Read the model definition and answer for the solid it produces. Units are mm, in the model's axes. Face numbers are marked on the shaded views. Coordinates: 2 decimals unless noted, no trailing zeros. Loops run counter-clockwise (first coordinate to the right, second up) from the corner with the lowest first, then second, coordinate; pieces in that order, holes last.
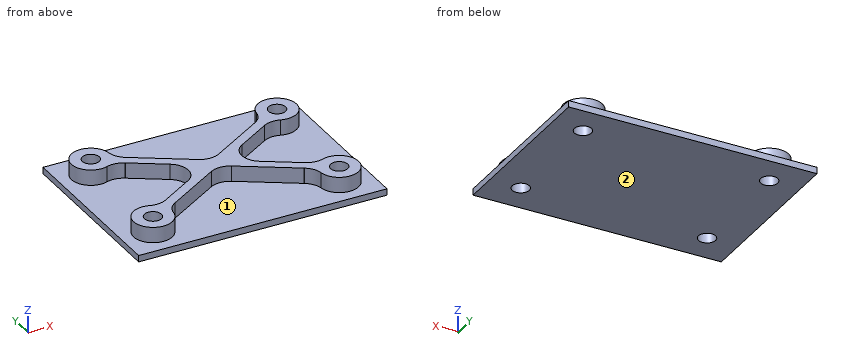
from build123d import *

# Parameters (mm, degrees)
F1_DEPTH = 3.175
F3_DEPTH = 7.62
F4_R     = 9.525
F5_R     = 4.2037
F6_DEPTH = 10.796


with BuildPart() as f1:
    # F0 (on Top) → F1 (new body)
    with BuildSketch(Plane.XY):
        with BuildLine():
            Line((15.24, -56.515), (15.24, 0))
            ThreePointArc((15.24, 0), (-10.7763073453, -10.7763073453), (0, 15.24))
            Line((0, 15.24), (-91.44, 15.24))
            ThreePointArc((-91.44, 15.24), (-80.6636926547, 10.7763073453), (-76.2, 0))
            ThreePointArc((-76.2, 0), (-91.44, -15.24), (-106.68, 0))
            Line((-106.68, 0), (-106.68, -56.515))
            ThreePointArc((-106.68, -56.515), (-91.44, -41.275), (-76.2, -56.515))
            ThreePointArc((-76.2, -56.515), (-80.6636926547, -67.2913073453), (-91.44, -71.755))
            Line((-91.44, -71.755), (0, -71.755))
            ThreePointArc((0, -71.755), (-10.7763073453, -45.7386926547), (15.24, -56.515))
        make_face()
        with BuildLine():
            ThreePointArc((-106.68, -56.515), (-102.2163073453, -67.2913073453), (-91.44, -71.755))
            ThreePointArc((-91.44, -71.755), (-80.6636926547, -67.2913073453), (-76.2, -56.515))
            ThreePointArc((-76.2, -56.515), (-91.44, -41.275), (-106.68, -56.515))
        make_face()
        with BuildLine():
            ThreePointArc((-76.2, 0), (-80.6636926547, 10.7763073453), (-91.44, 15.24))
            ThreePointArc((-91.44, 15.24), (-102.2163073453, 10.7763073453), (-106.68, 0))
            ThreePointArc((-106.68, 0), (-91.44, -15.24), (-76.2, 0))
        make_face()
        with BuildLine():
            ThreePointArc((0, 15.24), (-10.7763073453, -10.7763073453), (15.24, 0))
            ThreePointArc((15.24, 0), (10.7763073453, 10.7763073453), (0, 15.24))
        make_face()
        with BuildLine():
            ThreePointArc((0, -71.755), (10.7763073453, -67.2913073453), (15.24, -56.515))
            ThreePointArc((15.24, -56.515), (-10.7763073453, -45.7386926547), (0, -71.755))
        make_face()
        with BuildLine():
            Line((15.24, -71.755), (15.24, -56.515))
            ThreePointArc((15.24, -56.515), (10.7763073453, -67.2913073453), (0, -71.755))
            Line((0, -71.755), (15.24, -71.755))
        make_face()
        with BuildLine():
            Line((-106.68, -71.755), (-91.44, -71.755))
            ThreePointArc((-91.44, -71.755), (-102.2163073453, -67.2913073453), (-106.68, -56.515))
            Line((-106.68, -56.515), (-106.68, -71.755))
        make_face()
        with BuildLine():
            ThreePointArc((-106.68, 0), (-102.2163073453, 10.7763073453), (-91.44, 15.24))
            Line((-91.44, 15.24), (-106.68, 15.24))
            Line((-106.68, 15.24), (-106.68, 0))
        make_face()
        with BuildLine():
            ThreePointArc((0, 15.24), (10.7763073453, 10.7763073453), (15.24, 0))
            Line((15.24, 0), (15.24, 15.24))
            Line((15.24, 15.24), (0, 15.24))
        make_face()
    extrude(amount=-F1_DEPTH)

    # F2 (on face) → F3 (join)
    with BuildSketch(Plane.XY):
        with BuildLine():
            Line((-9.0970156165, -2.8231067769), (-14.056494823, -5.8883404532))
            ThreePointArc((-14.056494823, -5.8883404532), (-12.9637932823, -8.0123444592), (-11.5526371794, -9.9395258539))
            Line((-11.5526371794, -9.9395258539), (-6.593157973, -6.8742921776))
            ThreePointArc((-6.593157973, -6.8742921776), (8.1023708015, 5.007715287), (-9.0970156165, -2.8231067769))
        make_face()
        with BuildLine():
            ThreePointArc((-11.5526371794, -46.5754741461), (-12.9637932823, -48.5026555408), (-14.056494823, -50.6266595468))
            Line((-14.056494823, -50.6266595468), (-9.0970156165, -53.6918932231))
            ThreePointArc((-9.0970156165, -53.6918932231), (8.1023708015, -61.522715287), (-6.593157973, -49.6407078224))
            Line((-6.593157973, -49.6407078224), (-11.5526371794, -46.5754741461))
        make_face()
        with BuildLine():
            ThreePointArc((-77.383505177, -50.6266595468), (-78.4762067177, -48.5026555408), (-79.8873628206, -46.5754741461))
            Line((-79.8873628206, -46.5754741461), (-84.846842027, -49.6407078224))
            ThreePointArc((-84.846842027, -49.6407078224), (-99.5423708015, -61.522715287), (-82.3429843835, -53.6918932231))
            Line((-82.3429843835, -53.6918932231), (-77.383505177, -50.6266595468))
        make_face()
        with BuildLine():
            ThreePointArc((-82.3429843835, -2.8231067769), (-99.5423708015, 5.007715287), (-84.846842027, -6.8742921776))
            Line((-84.846842027, -6.8742921776), (-79.8873628206, -9.9395258539))
            ThreePointArc((-79.8873628206, -9.9395258539), (-78.4762067177, -8.0123444592), (-77.383505177, -5.8883404532))
            Line((-77.383505177, -5.8883404532), (-82.3429843835, -2.8231067769))
        make_face()
        with BuildLine():
            ThreePointArc((-77.383505177, -5.8883404532), (-78.4762067177, -8.0123444592), (-79.8873628206, -9.9395258539))
            Line((-79.8873628206, -9.9395258539), (-50.249292292, -28.2575))
            Line((-50.249292292, -28.2575), (-79.8873628206, -46.5754741461))
            ThreePointArc((-79.8873628206, -46.5754741461), (-78.4762067177, -48.5026555408), (-77.383505177, -50.6266595468))
            Line((-77.383505177, -50.6266595468), (-45.72, -31.0568542638))
            Line((-45.72, -31.0568542638), (-14.056494823, -50.6266595468))
            ThreePointArc((-14.056494823, -50.6266595468), (-12.9637932823, -48.5026555408), (-11.5526371794, -46.5754741461))
            Line((-11.5526371794, -46.5754741461), (-41.190707708, -28.2575))
            Line((-41.190707708, -28.2575), (-11.5526371794, -9.9395258539))
            ThreePointArc((-11.5526371794, -9.9395258539), (-12.9637932823, -8.0123444592), (-14.056494823, -5.8883404532))
            Line((-14.056494823, -5.8883404532), (-45.72, -25.4581457362))
            Line((-45.72, -25.4581457362), (-77.383505177, -5.8883404532))
        make_face()
    extrude(amount=F3_DEPTH)

    # F4
    f4_edges = [f1.edges().sort_by_distance(p)[0] for p in [
        (-45.72, -31.056854, 3.81),
        (-82.342984, -53.691893, 3.81),
        (-9.097016, -53.691893, 3.81),
        (-6.593158, -6.874292, 3.81),
        (-84.846842, -49.640708, 3.81),
        (-50.249292, -28.2575, 3.81),
        (-84.846842, -6.874292, 3.81),
        (-82.342984, -2.823107, 3.81),
        (-45.72, -25.458146, 3.81),
        (-9.097016, -2.823107, 3.81),
        (-41.190708, -28.2575, 3.81),
        (-6.593158, -49.640708, 3.81),
    ]]
    fillet(f4_edges, radius=F4_R)

    # F5 (on face) → F6 (cut, through all)
    with BuildSketch(Plane.XY.offset(7.62)):
        with Locations((0, -56.515)):
            Circle(F5_R)
        with Locations((-91.44, -56.515)):
            Circle(F5_R)
        with Locations((-91.44, 0)):
            Circle(F5_R)
        Circle(F5_R)
    extrude(amount=-F6_DEPTH, mode=Mode.SUBTRACT)


solid = f1.part
Item 1: A cutting plane is placed at B-B on x = -69. Determine the outline of the cut face in (y, z) (3 decimals).
Numbers:
outline: (-71.755, -3.175) - (15.24, -3.175) - (15.24, 0) - (-11.07, 0) - (-11.07, 7.62) - (-16.669, 7.62) - (-16.669, 0) - (-39.846, 0) - (-39.846, 7.62) - (-45.445, 7.62) - (-45.445, 0) - (-71.755, 0) - close
Item 2: A cutting plane is placed at C-C on z = 4.25. Give the number of separate pieces and of enclosed holes in the cut face, then the cut area to 3 significant figures.
Numbers:
separate pieces: 1
enclosed holes: 4
area: 1,890 mm2
Item 3: Given pin 1 (4 mm diameter, centred on x = -47.5, z = 5, fed in from +Y); pin 2 (5 mm diameter, centred on x = -32.5, z = 5.5, fed in from -Y), each flat-ended and moving along its own axis, determine where each tip first touches the part or whether it passes through.
Numbers:
pin 1: stops at y = -23
pin 2: stops at y = -40.77
Item 4: Find the intervals of material crossed by line 1 along Y through (x, z) = (0, -0.25) (3 decimals); line 2 along Y through (x, z) = (0, 5) (3 decimals); line 3 along Y through (x, z) = (-90.5, 6.5), in increasing order.
Numbers:
line 1: y = -71.755 to -60.719, -52.311 to -4.204, 4.204 to 15.24
line 2: y = -66.04 to -60.719, -52.311 to -46.99, -9.525 to -4.204, 4.204 to 9.525
line 3: y = -65.99 to -60.61, -52.42 to -47.04, -9.48 to -4.1, 4.1 to 9.48
Item 5: A cutting plane is placed at A-A on x = 0. Determine the outline of the cut face in (y, z) (3 decimals).
Numbers:
outline: (-71.755, -3.175) - (-60.719, -3.175) - (-60.719, 7.62) - (-66.04, 7.62) - (-66.04, 0) - (-71.755, 0) - close; (-52.311, -3.175) - (-4.204, -3.175) - (-4.204, 7.62) - (-9.525, 7.62) - (-9.525, 0) - (-46.99, 0) - (-46.99, 7.62) - (-52.311, 7.62) - close; (4.204, -3.175) - (15.24, -3.175) - (15.24, 0) - (9.525, 0) - (9.525, 7.62) - (4.204, 7.62) - close
Item 6: Determine the mould class of the marked faces 1 and 2 for opening direction X: released by +X, released by -X, zero draft, split by the parting line, or undercut.
Numbers:
face 1: undercut
face 2: zero draft
Item 7: A cutting plane is placed at D-D on x = -43. Determine the outline of the cut face in (y, z) (3 decimals).
Numbers:
outline: (-71.755, -3.175) - (15.24, -3.175) - (15.24, 0) - (-23.389, 0) - (-23.389, 7.62) - (-33.126, 7.62) - (-33.126, 0) - (-71.755, 0) - close
